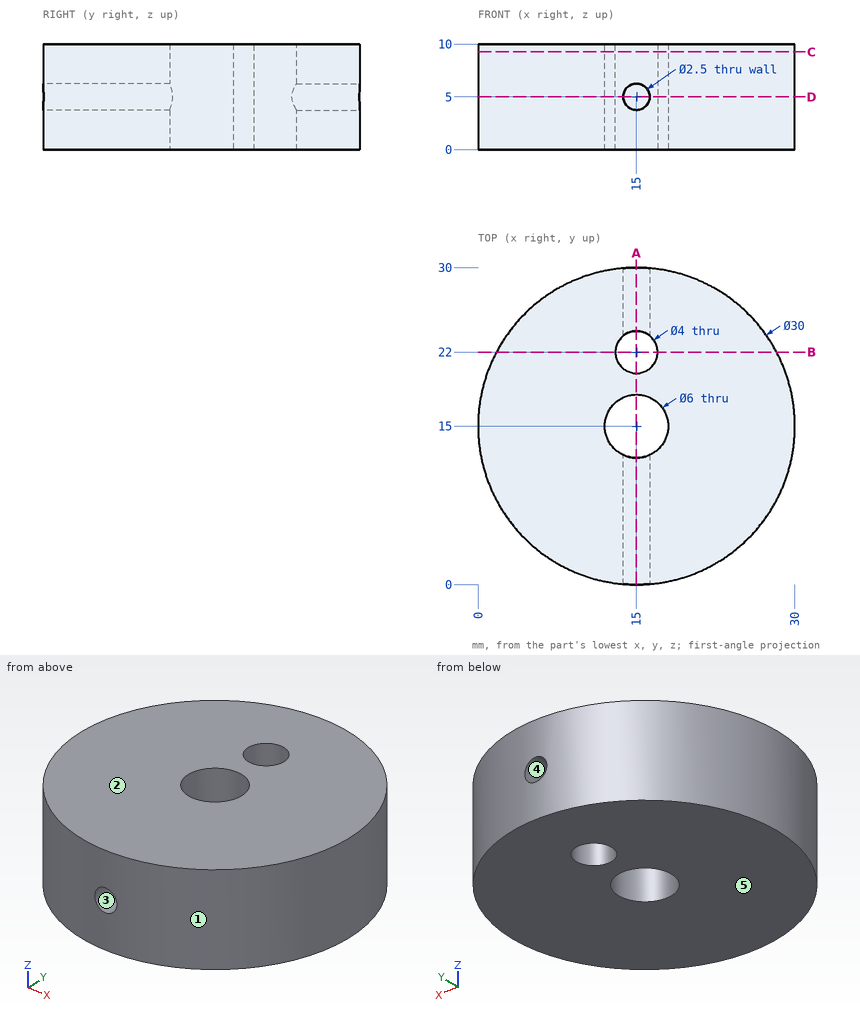
Geometry check sheet. Reference: drawing and pictorial views, mm from the part's lowest x, y, z. A direction names the side the tool comes from. Give positions to 0.01 mm unless a question says otherwise; leave off trailing zeros. Order: outer loops, then holes, each group sorted by start corner. A loop starts at its lowest first (then second) coordinate and runs counter-clockwise, first axis right, second up. Notation, with made-up numbers: M -7.5,-1 L 14.5,-1 A36 cw 14.5,38 Z; hole C 48,-7 d3. An arc over 180 degrees is marked long. Return JSON: item names as keys, results as strings. Group by question number.
1) Section check C-C on z = 9.25. Record the cut outline in (x, y).
2) Go/stop test with flat-tipped pins: pin 1 Ø4 at (x, z) = (12, 9) entering from -Y; pin 2 Ø6 at (y, z) = (19.5, 4) entering from -X; pin 3 Ø3 at (y, z) = (7.5, 8.5) entering from -X. Record where each tip stops, or that it passes through.
3) Scan lines: line 1 (Y direction, x = 15, z = 7.25); line 2 (Z direction, x = 15, y = 27); line 3 (X direction, y = 17, z = 8.75). Record each from-to range of solid material in increasing order.
4) Section check B-B on y = 22. Record the cut outline in (x, z), and give its area (3 significant figures).
5) Access from +Z, -Z, +X, -X, +Y, -Y to the whole of each face (thin tool, end or side, straight path). Record for the marked faces 4 and 5.
6) Section check D-D on z = 5. Record the cut outline in (x, y), and give its area (3 significant figures).
7) Mould release check, pull along X, two halves, no side actions. Record for the marked faces 1, 2 and 3: pulls with the +X half, pulls with the -X half, needs draft (parallel to the pull), parting line crosses it, or undercut.
8) Section check A-A on x = 15. Record the cut outline in (y, z), and give its area (3 significant figures).
Answer block:
{
 "1": {"outline": "C 15,15 d30; hole C 15,15 d6; hole C 15,22 d4"},
 "2": {"pin 1": "stops at y = 0.03", "pin 2": "stops at x = 0.08", "pin 3": "stops at x = 1.25"},
 "3": {"line 1": "y = 0 to 12, 18 to 20, 24 to 30", "line 2": "z = 0 to 3.75, 6.25 to 10", "line 3": "x = 0.13 to 12.76, 17.24 to 29.87"},
 "4": {"outline": "M 1.73,0 L 13,0 L 13,10 L 1.73,10 Z; M 17,0 L 28.27,0 L 28.27,10 L 17,10 Z", "area": "225 mm^2"},
 "5": {"face 4": "+Y", "face 5": "-Z, +X, -X, +Y, -Y"},
 "6": {"outline": "M 13.75,0.05 L 13.75,12.27 A3 cw long 16.25,12.27 L 16.25,0.05 A15 ccw 16.25,29.95 L 16.25,23.56 A2 cw long 13.75,23.56 L 13.75,29.95 A15 ccw Z", "area": "621 mm^2"},
 "7": {"face 1": "parting line crosses it", "face 2": "needs draft", "face 3": "undercut"},
 "8": {"outline": "M 0,0 L 12,0 L 12,3.75 L 0,3.75 Z; M 0,6.25 L 12,6.25 L 12,10 L 0,10 Z; M 18,0 L 20,0 L 20,10 L 18,10 Z; M 24,0 L 30,0 L 30,3.75 L 24,3.75 Z; M 24,6.25 L 30,6.25 L 30,10 L 24,10 Z", "area": "155 mm^2"}
}
